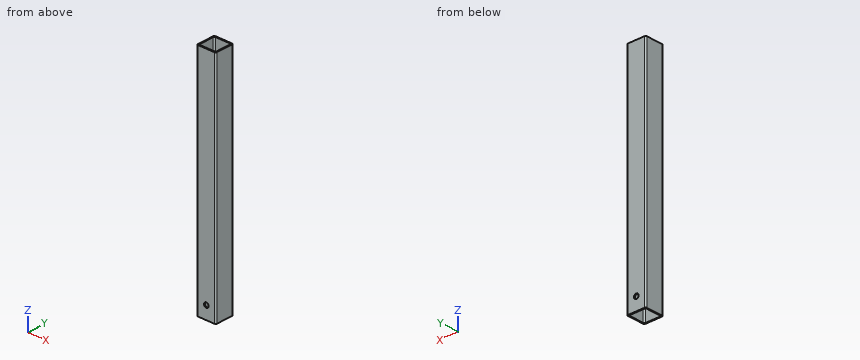
from build123d import *

# Parameters (mm, degrees)
SKETCH1_W           = 38.1
SKETCH1_H           = 38.1
SKETCH1_W_2         = 33.8836
SKETCH1_H_2         = 33.8836
BOSS_EXTRUDE1_DEPTH = 457.2
FILLET1_R           = 2.54
SKETCH2_R           = 4.7625
CUT_EXTRUDE1_DEPTH  = 460.180087221


with BuildPart() as part:
    # Sketch1 → Boss-Extrude1 (new body)
    with BuildSketch(Plane.XY):
        Rectangle(SKETCH1_W, SKETCH1_H)
        Rectangle(SKETCH1_W_2, SKETCH1_H_2, mode=Mode.SUBTRACT)
    extrude(amount=BOSS_EXTRUDE1_DEPTH)

    # Fillet1
    fillet1_edges = [part.edges().sort_by_distance(p)[0] for p in [
        (-16.9418, 16.9418, 228.6),
        (-16.9418, -16.9418, 228.6),
        (16.9418, -16.9418, 228.6),
        (16.9418, 16.9418, 228.6),
        (19.05, -19.05, 228.6),
        (-19.05, -19.05, 228.6),
        (-19.05, 19.05, 228.6),
        (19.05, 19.05, 228.6),
    ]]
    fillet(fillet1_edges, radius=FILLET1_R)

    # Sketch2 → Cut-Extrude1 (cut, through all)
    with BuildSketch(Plane(origin=(0, 19.05, 0), x_dir=(1, 0, 0), z_dir=(0, 1, 0))):
        with Locations(Location((0, -25.4, 0), (0, 0, 270))):
            Circle(SKETCH2_R)
    extrude(amount=-CUT_EXTRUDE1_DEPTH, mode=Mode.SUBTRACT)


solid = part.part
Build history of the part. All positions in model axes, mm. Round coordinates to 2 decimals unless told otherwise and drop trailing zeros. Write each loop counter-clockwise with the first axis right and the second up, starting at its lowest first coordinate (ties: lowest second). Pieces come first, ordered by that corner, then holes. Notation, with made-up numbers: (48, 4) - (57, 4) arc R18 ccw to (57, 16) - close; hole circle Ø10 at (-15.75, 15.25). An arc over 180 degrees is marked (long way). Use CSV: the item, a comma, the result in double quotes.
(1) Band-saw the part on D-D (z = 275). Write the cut outline in (x, y).
Response:
outline,"(-19.05, -16.51) arc R2.54 ccw to (-16.51, -19.05) - (16.51, -19.05) arc R2.54 ccw to (19.05, -16.51) - (19.05, 16.51) arc R2.54 ccw to (16.51, 19.05) - (-16.51, 19.05) arc R2.54 ccw to (-19.05, 16.51) - close; hole (-16.94, -14.4) arc R2.54 ccw to (-14.4, -16.94) - (14.4, -16.94) arc R2.54 ccw to (16.94, -14.4) - (16.94, 14.4) arc R2.54 ccw to (14.4, 16.94) - (-14.4, 16.94) arc R2.54 ccw to (-16.94, 14.4) - close"
(2) Band-saw the part on B-B (z = 25.4). Write the cut outline in (x, y), plus the area to 3 significant figures.
Response:
outline,"(-19.05, -16.51) arc R2.54 ccw to (-16.51, -19.05) - (-4.76, -19.05) - (-4.76, -16.94) - (-14.4, -16.94) arc R2.54 cw to (-16.94, -14.4) - (-16.94, 14.4) arc R2.54 cw to (-14.4, 16.94) - (-4.76, 16.94) - (-4.76, 19.05) - (-16.51, 19.05) arc R2.54 ccw to (-19.05, 16.51) - close; (4.76, -19.05) - (16.51, -19.05) arc R2.54 ccw to (19.05, -16.51) - (19.05, 16.51) arc R2.54 ccw to (16.51, 19.05) - (4.76, 19.05) - (4.76, 16.94) - (14.4, 16.94) arc R2.54 cw to (16.94, 14.4) - (16.94, -14.4) arc R2.54 cw to (14.4, -16.94) - (4.76, -16.94) - close"
area,"263 mm²"
(3) Band-saw the part on C-C (x = 0). Write the cut outline in (y, z), plus the area to 3 significant figures.
Response:
outline,"(-19.05, 0) - (-16.94, 0) - (-16.94, 20.64) - (-19.05, 20.64) - close; (-19.05, 30.16) - (-16.94, 30.16) - (-16.94, 457.2) - (-19.05, 457.2) - close; (16.94, 0) - (19.05, 0) - (19.05, 20.64) - (16.94, 20.64) - close; (16.94, 30.16) - (19.05, 30.16) - (19.05, 457.2) - (16.94, 457.2) - close"
area,"1,890 mm²"
(4) Band-saw the part on A-A (y = 4.5). Write the cut outline in (x, z), plus the area to 3 significant figures.
Response:
outline,"(-19.05, 0) - (-16.94, 0) - (-16.94, 457.2) - (-19.05, 457.2) - close; (16.94, 0) - (19.05, 0) - (19.05, 457.2) - (16.94, 457.2) - close"
area,"1,930 mm²"
(5) Wall check: line 1 (Y direction, x = 10.5, z = 28); line 2 (X direction, y = -17, z = 25). Give the ranges that are in metal, low to high.
Response:
line 1,"-19.05 to -16.94, 16.94 to 19.05"
line 2,"-19 to -4.75, 4.75 to 19"
